Could you check a few things on this model? Use its own coordinates, in mm. A direction names the side the tool comes from. Round coordinates to 2 decimals unless told otherwise and drop trailing zeros. Loops run counter-clockwise (first coordinate to the right, second up) from the corner with the lowest first, then second, coordinate; pieces in that order, holes last.
from build123d import *

# Parameters (mm, degrees)
EXTRUDE_1_DEPTH     = 35
SKETCH_2_W          = 48
SKETCH_2_H          = 14
CUT_EXTRUDE_1_DEPTH = 4
SKETCH_3_R          = 2
CUT_EXTRUDE_2_DEPTH = 19


with BuildPart() as part:
    # Эскиз1 → Бобышка-Вытянуть1 (new body)
    with BuildSketch(Plane.XY):
        with BuildLine():
            Line((0, 0), (9, 0))
            ThreePointArc((9, 0), (11.121320344, 0.878679656), (12, 3))
            Line((12, 3), (12, 15))
            ThreePointArc((12, 15), (12.292893219, 15.707106781), (13, 16))
            Line((13, 16), (35, 16))
            ThreePointArc((35, 16), (35.707106781, 15.707106781), (36, 15))
            Line((36, 15), (36, 3))
            ThreePointArc((36, 3), (36.878679656, 0.878679656), (39, 0))
            Line((39, 0), (48, 0))
            Line((48, 0), (48, 2))
            Line((48, 2), (39, 2))
            ThreePointArc((39, 2), (38.292893219, 2.292893219), (38, 3))
            Line((38, 3), (38, 15))
            ThreePointArc((38, 15), (37.121320344, 17.121320344), (35, 18))
            Line((35, 18), (13, 18))
            ThreePointArc((13, 18), (10.878679656, 17.121320344), (10, 15))
            Line((10, 15), (10, 3))
            ThreePointArc((10, 3), (9.707106781, 2.292893219), (9, 2))
            Line((9, 2), (0, 2))
            Line((0, 2), (0, 0))
        make_face()
    extrude(amount=EXTRUDE_1_DEPTH)

    # Эскиз2 → Вырез-Вытянуть1 (cut)
    with BuildSketch(Plane(origin=(0, 18, 0), x_dir=(1, 0, 0), z_dir=(0, 1, 0))):
        with Locations((24, -7)):
            Rectangle(SKETCH_2_W, SKETCH_2_H)
    extrude(amount=-CUT_EXTRUDE_1_DEPTH, mode=Mode.SUBTRACT)

    # Эскиз3 → Вырез-Вытянуть2 (cut, through all)
    with BuildSketch(Plane(origin=(0, 18, 0), x_dir=(1, 0, 0), z_dir=(0, 1, 0))):
        with Locations((24, -19)):
            Circle(SKETCH_3_R)
        with Locations((24, -27)):
            Circle(SKETCH_3_R)
        with Locations((5, -30)):
            Circle(SKETCH_3_R)
        with Locations((5, -5)):
            Circle(SKETCH_3_R)
        with Locations((43, -30)):
            Circle(SKETCH_3_R)
        with Locations((43, -5)):
            Circle(SKETCH_3_R)
    extrude(amount=-CUT_EXTRUDE_2_DEPTH, mode=Mode.SUBTRACT)


solid = part.part
Item 1: For faces 1 (the flat face through (38, 9, 17)), 2 (the flat face through (37, 14, 7)), 3 (the flat face through (12, 9, 17)), 4 (the flat face through (10, 9, 17)), which set-ups out of +Z, -Z, +X, -X, +Y, -Y let a thin tool reach every point of the face, with its end or its side?
Results list:
face 1: +Z, -Z, +X, +Y
face 2: -Z, +X, -X, +Y
face 3: +Z, -Z, -Y
face 4: +Z, -Z, -X, +Y
Item 2: If we section it at C-C, the plane y = 4: Please give me the cut outline in (x, z).
Results list:
outline: (10, 0) - (12, 0) - (12, 35) - (10, 35) - close; (36, 0) - (38, 0) - (38, 35) - (36, 35) - close
Item 3: Will these pins go through, and if not, where does the flat tip stop? pin 1 (10 mm diameter, centred on y = 13.5, z = 26.5, fed in from -X); pin 2 (1 mm diameter, centred on x = 37, z = 8, fed in from +Y); pin 3 (6.5 mm diameter, centred on x = 24, z = 19, fed in from -Y).
Results list:
pin 1: stops at x = 10
pin 2: stops at y = 14
pin 3: stops at y = 16
Item 4: If we section it at B-B, the plane z = 7.5: Please give me the cut outline in (x, y).
Results list:
outline: (0, 0) - (9, 0) arc R3 ccw to (12, 3) - (12, 14) - (10, 14) - (10, 3) arc R1 cw to (9, 2) - (0, 2) - close; (36, 3) arc R3 ccw to (39, 0) - (48, 0) - (48, 2) - (39, 2) arc R1 cw to (38, 3) - (38, 14) - (36, 14) - close
Item 5: If we section it at A-A, the plane x = 24: Please give me the cut outline in (y, z).
Results list:
outline: (16, 14) - (18, 14) - (18, 17) - (16, 17) - close; (16, 21) - (18, 21) - (18, 25) - (16, 25) - close; (16, 29) - (18, 29) - (18, 35) - (16, 35) - close
Item 6: If I drill on line 1 along Z through (x, y) = (24, 16.6); line 2 along Z through (x, y) = (5, 1.3); line 3 along X through (y, z) = (1, 5), over which ranges is the centre line in solid material (lowest first)?
Results list:
line 1: z = 14 to 17, 21 to 25, 29 to 35
line 2: z = 0 to 3, 7 to 28, 32 to 35
line 3: x = 0 to 3, 7 to 11.24, 36.76 to 41, 45 to 48
Item 7: We'd pull the mould along Z, two halves only. Please class faces 5 (the cylindrical face through (41, 1, 5)), 6 (the flat face through (0, 1, 17)), 7 (the flat face through (23.8, 16.5, 14)): released by +Z, released by -Z, zero draft, split by the parting line, or undercut.
Results list:
face 5: undercut
face 6: zero draft
face 7: released by -Z
Item 8: If we section it at D-D, the plane z = 30: Please give me the cut outline in (x, y), then the cut area to 3 significant figures.
Results list:
outline: (0, 0) - (3, 0) - (3, 2) - (0, 2) - close; (7, 0) - (9, 0) arc R3 ccw to (12, 3) - (12, 15) arc R1 cw to (13, 16) - (35, 16) arc R1 cw to (36, 15) - (36, 3) arc R3 ccw to (39, 0) - (41, 0) - (41, 2) - (39, 2) arc R1 cw to (38, 3) - (38, 15) arc R3 ccw to (35, 18) - (13, 18) arc R3 ccw to (10, 15) - (10, 3) arc R1 cw to (9, 2) - (7, 2) - close; (45, 0) - (48, 0) - (48, 2) - (45, 2) - close
area: 137 mm2
